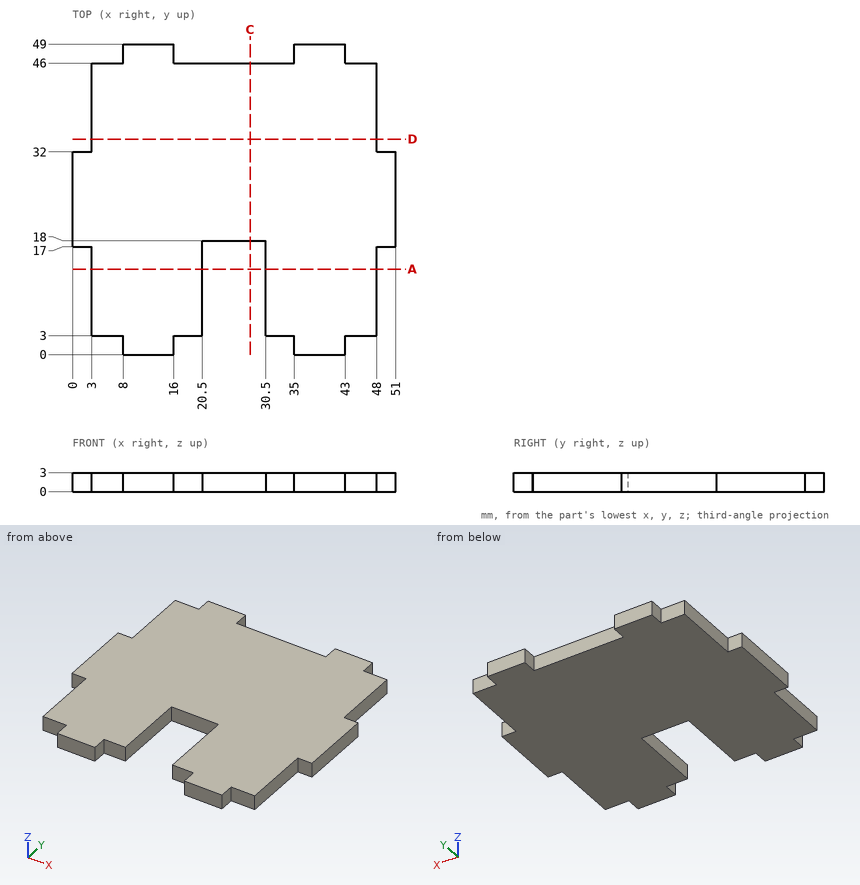
Part print with two shaded views. Sizes in mm from the minimum x, y, z corner. Coordinates: 2 decimals unless noted, no trailing zeros. Write each loop counter-clockwise with the first axis right and the second up, starting at its lowest first coordinate (ties: lowest second). Pieces come first, ordered by that corner, then holes.
(1) Pin check, flat tips, straight feed: pin 1 Ø0.9 at (y, z) = (1.5, 2) entering from -X; pin 2 Ø1.5 at (y, z) = (13, 1) entering from -X; pin 3 Ø1.5 at (x, z) = (21, 1) entering from +Y. Stop position of each tip, or through.
(2) Cut at A-A on y = 13.5. List the corners of the cut face in (x, z).
(3) Cut at C-C on x = 28. List the corners of the cut face in (y, z).
(4) Drill centre lines: line 1 (X direction, y = 15.5, z = 0.6); line 2 (Y direction, x = 28, z = 0.85); line 3 (Y direction, x = 33, z = 0.35). Where is each one in solid material? Low to high.
(5) Cut at D-D on y = 34. List the corners of the cut face in (x, z), and give its area (3 significant figures).
Working result:
1. pin 1: stops at x = 8
1. pin 2: stops at x = 3
1. pin 3: stops at y = 46
2. outline: (3, 0) - (20.5, 0) - (20.5, 3) - (3, 3) - close; (30.5, 0) - (48, 0) - (48, 3) - (30.5, 3) - close
3. outline: (18, 0) - (46, 0) - (46, 3) - (18, 3) - close
4. line 1: x = 3 to 20.5, 30.5 to 48
4. line 2: y = 18 to 46
4. line 3: y = 3 to 46
5. outline: (3, 0) - (48, 0) - (48, 3) - (3, 3) - close
5. area: 135 mm2
